Check sheet for the drawn part. Datum: minimum x, y, z corner. Units: mm. Round coordinates to 2 decimals unless told otherwise and drop trailing zeros. Loops run counter-clockwise (first coordinate to the right, second up) from the corner with the lowest first, then second, coordinate; pieces in that order, holes last.
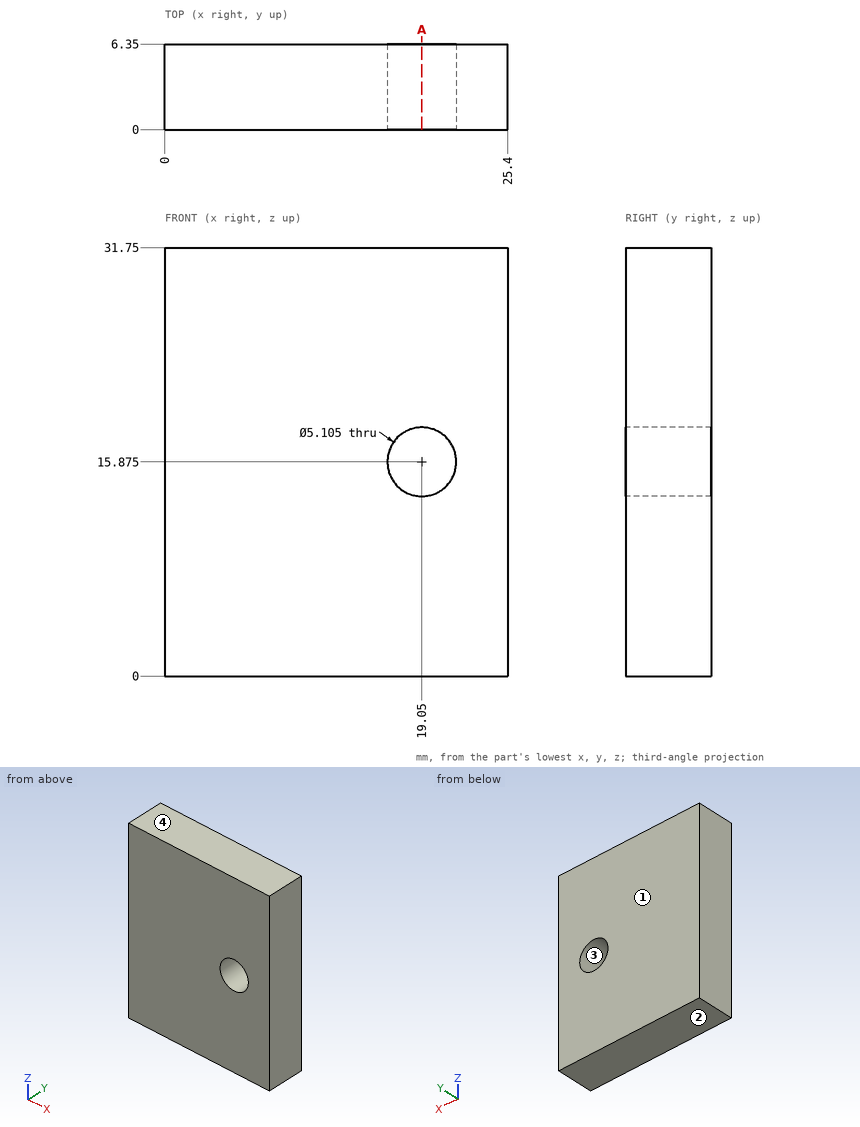
1) Mould release check, pull along Z, two halves, no side actions. Record for the marked faces 1, 2, 3 and 4: +Z half, -Z half, draft (parallel to the pull), parting line (faces both ways), or undercut.
Report:
face 1: draft
face 2: -Z half
face 3: undercut
face 4: +Z half
2) Gauge pin test, flat end, axial feed: pin 1 (4 mm diameter, centred on x = 15.5, z = 9, fed in from -Y). Record the tip position at first contact, or that the pin passes through.
Report:
pin 1: stops at y = 0
3) Sectioned sample at A-A, the plane x = 19.05. Record the cut outline in (y, z).
Report:
outline: (0, 0) - (6.35, 0) - (6.35, 13.32) - (0, 13.32) - close; (0, 18.43) - (6.35, 18.43) - (6.35, 31.75) - (0, 31.75) - close
